from build123d import *

# Parameters (mm, degrees)
SKETCH1_W           = 304.8
SKETCH1_H           = 152.4
SKETCH1_R           = 41.275
SKETCH1_R_2         = 3.81
SKETCH1_R_3         = 3.302
BOSS_EXTRUDE1_DEPTH = 2.54
SKETCH2_R           = 28.575
CUT_EXTRUDE1_DEPTH  = 3.54


with BuildPart() as part:
    # Sketch1 → Boss-Extrude1 (new body)
    with BuildSketch(Plane(origin=(0, 0, 0), x_dir=(1, 0, 0), z_dir=(0, 1, 0))):
        Rectangle(SKETCH1_W, SKETCH1_H)
        with Locations((-100.803124952, 0)):
            Circle(SKETCH1_R, mode=Mode.SUBTRACT)
        with Locations((101.6, 0)):
            Circle(SKETCH1_R, mode=Mode.SUBTRACT)
        with Locations((146.05, 47.625)):
            Circle(SKETCH1_R_2, mode=Mode.SUBTRACT)
        with Locations((76.2, 69.85)):
            Circle(SKETCH1_R_3, mode=Mode.SUBTRACT)
        with Locations((-146.05, 47.625)):
            Circle(SKETCH1_R_2, mode=Mode.SUBTRACT)
        with Locations((-146.05, -47.625)):
            Circle(SKETCH1_R_2, mode=Mode.SUBTRACT)
        with Locations((-76.2, -69.85)):
            Circle(SKETCH1_R_3, mode=Mode.SUBTRACT)
        with Locations((76.2, -69.85)):
            Circle(SKETCH1_R_3, mode=Mode.SUBTRACT)
        with Locations((146.05, -47.625)):
            Circle(SKETCH1_R_2, mode=Mode.SUBTRACT)
        with Locations((0, -69.85)):
            Circle(SKETCH1_R_2, mode=Mode.SUBTRACT)
        with Locations((-76.2, 69.85)):
            Circle(SKETCH1_R_3, mode=Mode.SUBTRACT)
        with Locations((0, 69.85)):
            Circle(SKETCH1_R_2, mode=Mode.SUBTRACT)
    extrude(amount=BOSS_EXTRUDE1_DEPTH)

    # Sketch2 → Cut-Extrude1 (cut, through all)
    with BuildSketch(Plane(origin=(0, 2.54, 0), x_dir=(1, 0, 0), z_dir=(0, 1, 0))):
        with Locations((-38.1, 40.8686)):
            Circle(SKETCH2_R)
    extrude(amount=-CUT_EXTRUDE1_DEPTH, mode=Mode.SUBTRACT)


solid = part.part
Build history of the part. All positions in model axes, mm. Round coordinates to 2 decimals unless told otherwise and drop trailing zeros. Write each loop counter-clockwise with the first axis right and the second up, starting at its lowest first coordinate (ties: lowest second). Pieces come first, ordered by that corner, then holes. Notation, with made-up numbers: M 37.5,33.5 L 66.5,33.5 A21 cw 66.5,44.5 Z; hole C 2,52.25 d3. An arc over 180 degrees is marked long. Answer as a JSON object with one key per item and string values. Group by question number.
(1) Cut at D-D (z = 31.5). Give the cut face in (x, y), and give its area (3 significant figures).
(2) Mould opens along Z. For faces 1 (the cylindrical face through (73.766, 1.252, 67.618)), 2 (the flat face through (-2, 2.54, -1)) say: pulls with the +Z half, pulls with the -Z half, needs draft (parallel to the pull), parting line crosses it, or undercut.
(3) Drill centre lines: L1, parallel to X at y = 1.4, z = -69.85; L2, parallel to X at y = 0.8, z = -50; L3, parallel to Z at x = 101, y = 0.85. Where is each one in solid material? Low to high.
(4) Flat gauge pin, fed straight in: pin 1 (10 mm diameter, centred on x = -146.05, z = 47.625, fed in from +Y). Where does the tip first touch, or does it go through?
(5) Cut at B-B (x = 101.6). Give the cut face in (y, z) (3 decimals).
(6) Cut at C-C (x = 146.05). Give the cut face in (y, z) (3 decimals).
(7) Cut at A-A (z = 69.85). Give the cut face in (x, y), and give its area (3 significant figures).
Responses:
{
 "1": {"outline": "M -152.4,0 L -127.47,0 L -127.47,2.54 L -152.4,2.54 Z; M -74.13,0 L 74.93,0 L 74.93,2.54 L -74.13,2.54 Z; M 128.27,0 L 152.4,0 L 152.4,2.54 L 128.27,2.54 Z", "area": "503 mm2"},
 "2": {"face 1": "undercut", "face 2": "needs draft"},
 "3": {"L1": "x = -152.4 to -79.5, -72.9 to -3.81, 3.81 to 72.9, 79.5 to 152.4", "L2": "x = -152.4 to -149.03, -143.07 to -65.18, -11.02 to 143.07, 149.03 to 152.4", "L3": "z = -76.2 to -41.27, 41.27 to 76.2"},
 "4": {"pin 1": "stops at y = 2.54"},
 "5": {"outline": "M 0,-76.2 L 2.54,-76.2 L 2.54,-41.275 L 0,-41.275 Z; M 0,41.275 L 2.54,41.275 L 2.54,76.2 L 0,76.2 Z"},
 "6": {"outline": "M 0,-76.2 L 2.54,-76.2 L 2.54,-51.435 L 0,-51.435 Z; M 0,-43.815 L 2.54,-43.815 L 2.54,43.815 L 0,43.815 Z; M 0,51.435 L 2.54,51.435 L 2.54,76.2 L 0,76.2 Z"},
 "7": {"outline": "M -152.4,0 L -79.5,0 L -79.5,2.54 L -152.4,2.54 Z; M -72.9,0 L -3.81,0 L -3.81,2.54 L -72.9,2.54 Z; M 3.81,0 L 72.9,0 L 72.9,2.54 L 3.81,2.54 Z; M 79.5,0 L 152.4,0 L 152.4,2.54 L 79.5,2.54 Z", "area": "721 mm2"}
}
